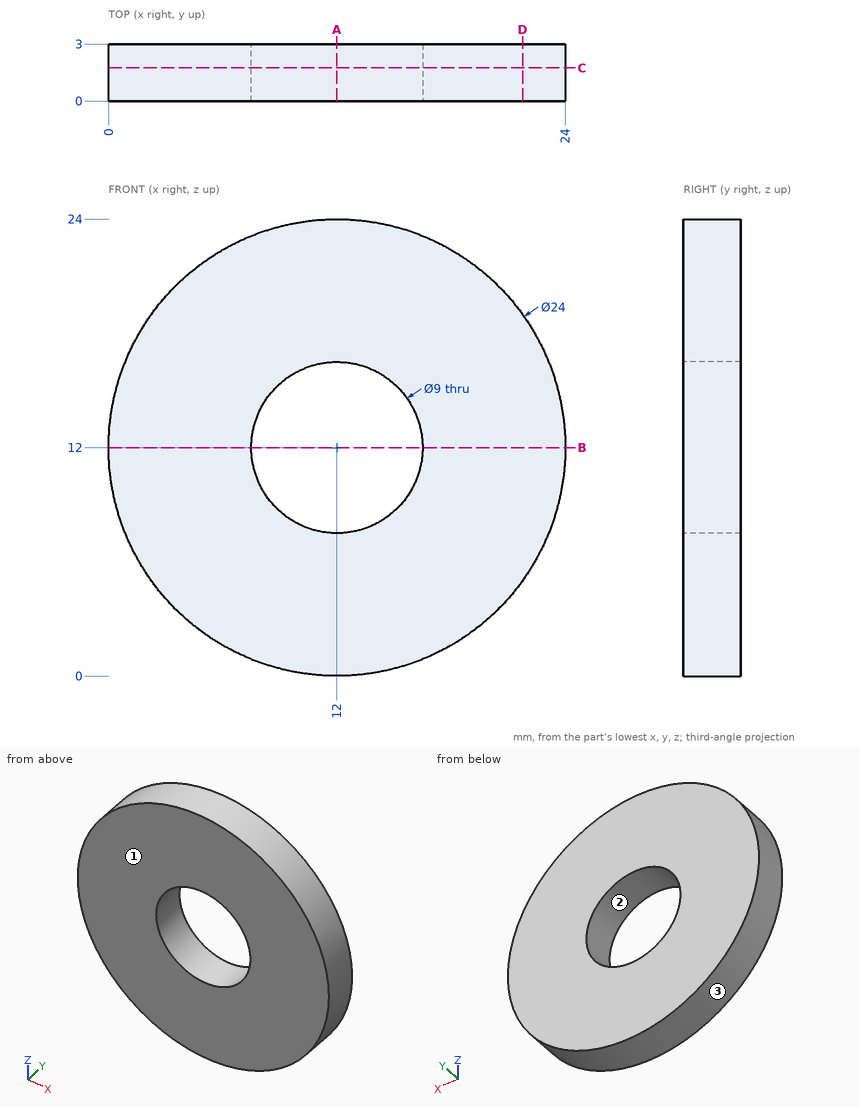
The figure shows three views and two pictorial views of one solid part (mm, origin at its lowest corner). Answer the questions. Coordinates: 2 decimals unless noted, no trailing zeros. Order: outer loops, then holes, each group sorted by start corner. A loop starts at its lowest first (then second) coordinate and runs counter-clockwise, first axis right, second up.
Q1. Consider line 1 (Z direction, x = 12, y = 2.25); line 2 (Z direction, x = 16, y = 2.2); line 3 (X direction, y = 1.85, z = 14). Determine where each line is inside the solid, lowest interval first.
Q2. A cutting plane is placed at A-A, the plane x = 12. Write down the section's boundary in (y, z).
Q3. Given P1, Ø1, axis at y = 2, z = 10.5, coming from the +X side; P2, Ø1, axis at y = 1.5, z = 20, coming from the +X side, each flat-ended and moving along its own axis, determine where each tip first touches the part or whether it passes through.
Q4. For a pull along X with two mould halves and no side action, classify the marked faces 1, 2 and 3 as pulls with the +X half, pulls with the -X half, needs draft (parallel to the pull), parting line crosses it, or undercut.
Q5. A cutting plane is placed at B-B, the plane z = 12. Write down the section's boundary in (x, y), and give its area (3 significant figures).
Q6. A cutting plane is placed at D-D, the plane x = 21.75. Write down the section's boundary in (y, z), and give its area (3 significant figures).
Q7. A cutting plane is placed at C-C, the plane y = 1.75. Write down the section's boundary in (x, z), and give its area (3 significant figures).
Answers follow:
1. line 1: z = 0 to 7.5, 16.5 to 24
1. line 2: z = 0.69 to 9.94, 14.06 to 23.31
1. line 3: x = 0.17 to 7.97, 16.03 to 23.83
2. outline: (0, 0) - (3, 0) - (3, 7.5) - (0, 7.5) - close; (0, 16.5) - (3, 16.5) - (3, 24) - (0, 24) - close
3. P1: stops at x = 23.96
3. P2: stops at x = 21.37
4. face 1: needs draft
4. face 2: undercut
4. face 3: parting line crosses it
5. outline: (0, 0) - (7.5, 0) - (7.5, 3) - (0, 3) - close; (16.5, 0) - (24, 0) - (24, 3) - (16.5, 3) - close
5. area: 45.0 mm2
6. outline: (0, 5) - (3, 5) - (3, 19) - (0, 19) - close
6. area: 42.0 mm2
7. outline: circle Ø24 at (12, 12); hole circle Ø9 at (12, 12)
7. area: 389 mm2
